For this review, use the dimensioned drawing (mm, ordinates from the lowest corner) and the shaded views. Give positions to 0.01 mm unless a question says otherwise; leave off trailing zeros. Order: outer loops, then holes, each group sorted by start corner. A loop starts at its lowest first (then second) coordinate and runs counter-clockwise, first axis right, second up.
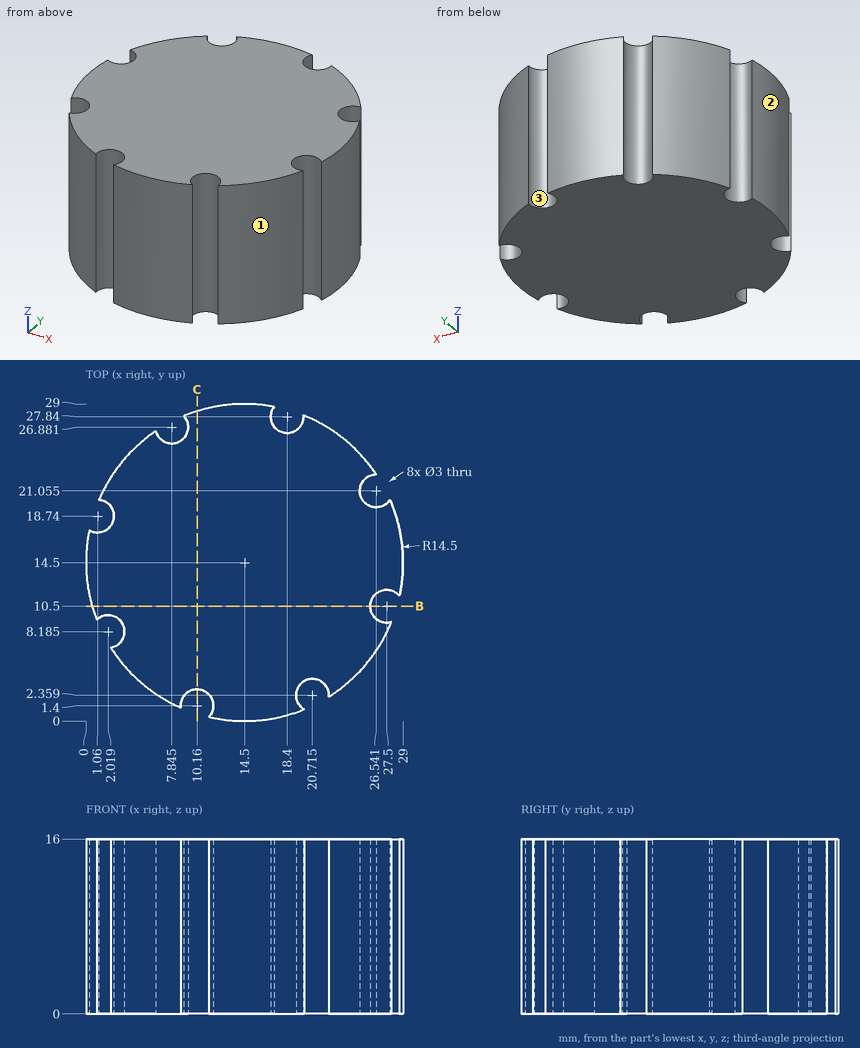
1. For pin 1 (2.5 mm diameter, centred on x = 1.06, y = 18.74, fed in from +Z); pin 2 (3 mm diameter, centred on x = 9, z = 6, fed in from +Y), all flat-tipped, find the tip position at first contact; note any pin that passes through.
Recorded:
pin 1: passes through
pin 2: stops at y = 28.44
2. For line 1 along Y through (x, z) = (2.75, 9) (1 decimal); line 2 along X through (y, z) = (27.5, 5.5) (1 decimal); line 3 along X through (y, z) = (3.5, 9.25) (1 decimal), list the stretches that pass through material, from the lowest coordinate up.
Recorded:
line 1: y = 6 to 6.9, 9.5 to 23
line 2: x = 9.2 to 16.9, 19.9 to 20.9
line 3: x = 5.1 to 19.7, 21.7 to 23.9
3. Take a section at B-B (y = 10.5). State the section outline as (x, z) points, then the cut area to 3 significant figures.
Recorded:
outline: (0.56, 0) - (26, 0) - (26, 16) - (0.56, 16) - close
area: 407 mm2
4. Take a section at C-C (x = 10.16). State the section outline as (y, z) points (1 decimal), then the cut area to 3 significant figures.
Recorded:
outline: (2.9, 0) - (28.3, 0) - (28.3, 16) - (2.9, 16) - close
area: 407 mm2
5. Draft analysis for pull direction Y (two halves, no side actions). For the marked faces 1, 2 and 3, state which applies: pulls with the +Y half, pulls with the -Y half, needs draft (parallel to the pull), parting line crosses it, or undercut.
Recorded:
face 1: pulls with the -Y half
face 2: parting line crosses it
face 3: undercut
